Job drawing, mm, ordinate dimensions from the low corner. One solid piece. A direction names the side the tool comes from. Give positions to 0.01 mm unless a question says otherwise; leave off trailing zeros. Loops run counter-clockwise (first coordinate to the right, second up) from the corner with the lowest first, then second, coordinate; pieces in that order, holes last. Notation, with made-up numbers: (11.25, 25.5) - (50.25, 25.5) arc R18 ccw to (50.25, 34.5) - close; hole circle Ø5 at (78.5, -29.75). An arc over 180 degrees is marked (long way). Use a Markdown table: item, result.
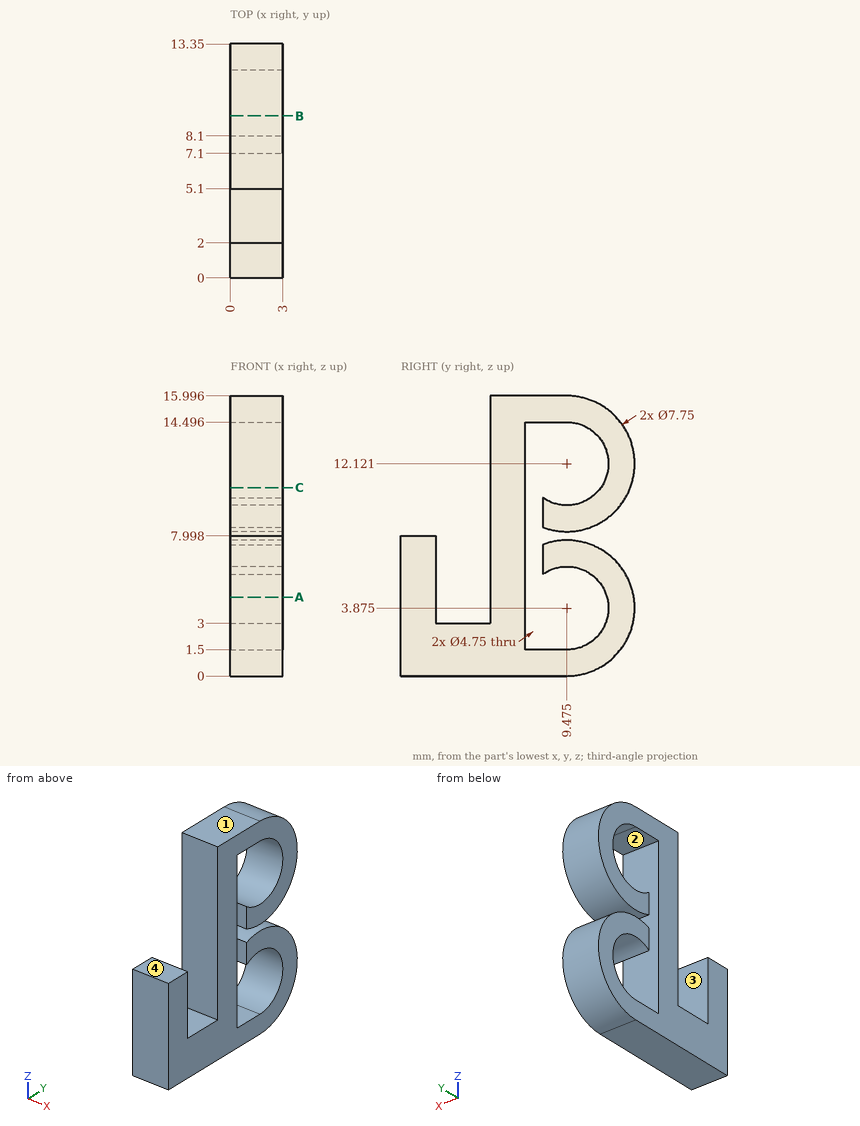
(1) Pin check, flat tips, straight feed: P1, Ø0.9, axis at x = 1, z = 5, coming from the +Y side; P2, Ø0.6, axis at x = 2, y = 1, coming from the +Z side; P3, Ø0.8, axis at x = 2, z = 9.5, coming from the -Y side. Stop position of each tip, or through.
Computed:
| item | result |
|---|---|
| P1 | y = 13.29 |
| P2 | z = 8 |
| P3 | y = 5.1 |
(2) Slice it at A-A, the plane z = 4.5. Write the cut outline in (x, y), plus the area to 3 significant figures.
Computed:
| item | result |
|---|---|
| outline | (0, 0) - (3, 0) - (3, 2) - (0, 2) - close; (0, 5.1) - (3, 5.1) - (3, 7.1) - (0, 7.1) - close; (0, 11.77) - (3, 11.77) - (3, 13.3) - (0, 13.3) - close |
| area | 16.6 mm² |
(3) Slice it at C-C, the plane z = 10.75. Write the cut outline in (x, y) (1 decimal).
Computed:
| item | result |
|---|---|
| outline | (0, 5.1) - (3, 5.1) - (3, 7.1) - (0, 7.1) - close; (0, 11.4) - (3, 11.4) - (3, 13.1) - (0, 13.1) - close |
(4) 3-axis set-ups, long thin cutter, end or side, ignore diameter. For the marked faces 1, 2, 3 and 4: which of +Z, -Z, +X, -X, +Y, -Y reach the whole face in a straight line?
Computed:
| item | result |
|---|---|
| face 1 | +Z, +X, -X, +Y, -Y |
| face 2 | +X, -X |
| face 3 | +Z, +X, -X |
| face 4 | +Z, +X, -X, -Y |
(5) Slice it at B-B, the plane y = 9.25. Write the cut outline in (x, z).
Computed:
| item | result |
|---|---|
| outline | (0, 0) - (3, 0) - (3, 1.5) - (0, 1.5) - close; (0, 6.24) - (3, 6.24) - (3, 7.74) - (0, 7.74) - close; (0, 8.25) - (3, 8.25) - (3, 9.76) - (0, 9.76) - close; (0, 14.5) - (3, 14.5) - (3, 16) - (0, 16) - close |
(6) Drill centre lines: probe 1 along Y at (x, z) = (1.15, 12.25); probe 2 along Z at (x, y) = (0.8, 8.5) (1 decimal); probe 3 along Z at (x, y) = (2.05, 9) (1 decimal). Where is each one in solid material? Low to high. Write a range as [from, to].
Computed:
| item | result |
|---|---|
| probe 1 | [5.1, 7.1], [11.85, 13.35] |
| probe 2 | [0, 1.5], [6, 7.6], [8.4, 10], [14.5, 16] |
| probe 3 | [0, 1.5], [6.2, 7.7], [8.3, 9.8], [14.5, 16] |
